Solid Edge part; units mm, degrees
sketch "Sketch1" plane through (0, 0, 0) normal (0, 0, 1) x (1, 0, 0)
  line L0 (-23, -6) -> (23, -6)
  arc A0 (23, 6) -> (23, -6) centre (23, 0) cw
  line L1 (23, 6) -> (-23, 6)
  arc A1 (-23, -6) -> (-23, 6) centre (-23, 0) cw
extrude "Protrusion1" add sketch "Sketch1" against normal blind 0.5
sketch "Sketch2" plane through (0, 0, 0) normal (0, 0, 1) x (1, 0, 0)
  circle A0 centre (26, 0) radius 1.5
extrude "ExtrudedProtrusion_2" add sketch "Sketch2" along normal blind 1
sketch "Sketch3" plane through (0, 0, 0) normal (0, 0, 1) x (1, 0, 0)
  line L0 (-12, -1.5) -> (20, -1.5)
  line L1 (20, -1.5) -> (20, 1.5)
  line L2 (20, 1.5) -> (-12, 1.5)
  line L3 (-12, -1.5) -> (-12, 1.5)
extrude "ExtrudedCutout_1" cut sketch "Sketch3" against normal blind 0.5
sketch "Sketch4" plane through (0, 0, 0) normal (0, 0, 1) x (1, 0, 0)
  circle A0 centre (-23, 3) radius 1
extrude "ExtrudedCutout_2" cut sketch "Sketch4" against normal blind 0.5
sketch "Sketch5" plane through (0, 0, 0) normal (0, 0, 1) x (1, 0, 0)
  circle A0 centre (-23, -3) radius 1
extrude "ExtrudedCutout_3" cut sketch "Sketch5" against normal blind 0.5
sketch "Sketch6" plane through (0, 0, 0) normal (0, 0, 1) x (1, 0, 0)
  circle A0 centre (23, 3) radius 1
extrude "ExtrudedCutout_4" cut sketch "Sketch6" against normal blind 0.5
sketch "Sketch7" plane through (0, 0, 0) normal (0, 0, 1) x (1, 0, 0)
  circle A0 centre (23, -3) radius 1
extrude "ExtrudedCutout_5" cut sketch "Sketch7" against normal blind 0.5
The listing builds one solid part. Answer for the finished solid, in the listing's coordinates (mm). Round coordinates to 2 decimals unless told otherwise and drop trailing zeros. Write each loop counter-clockwise with the first axis right and the second up, starting at its lowest first coordinate (ties: lowest second). Pieces come first, ordered by that corner, then holes. Notation, with made-up numbers: M 85.5,-33 L 97.5,-33 A9 cw 97.5,-29 Z; hole C 79.5,66 d5. An arc over 180 degrees is marked long. Write each question's results on one line, items separated by ' | '. Start each with the question number.
Item 1: Find section C-C on y = -0.5. Write down the section's boundary in (x, z), and give its area (3 significant figures).
Item 2: The mould has two halves that part along X. Classify faces 1 (the flat face through (0, 3, 0)), 2 (the cylindrical face through (-24, -3, -0.2)), 3 (the cylindrical face through (24.5, -0.07, 0.49)): +X half, -X half, draft (parallel to the pull), parting line (faces both ways), or undercut.
Item 3: Given pin 1 Ø6 at (x, y) = (19.5, 2.5) entering from +Z; pin 2 Ø1.8 at (x, y) = (23, 3) entering from -Z, each flat-ended and moving along its own axis, determine where each tip first touches the part or whether it passes through.
Item 4: Find section D-D on y = 3. Write down the section's boundary in (x, z).
Item 5: Find section A-A on x = 0. Write down the section's boundary in (y, z).
Item 6: Find section B-B on z = -0.25. Write down the section's boundary in (x, y), and give its area (3 significant figures).
Item 7: Straight lines are drawn through the part: probe 1 along Y at (x, z) = (-23, -0.1); probe 2 along Y at (x, z) = (3, -0.15); probe 3 along Z at (x, y) = (13, 3). For each, find the intervals that lie inside material, in ascending order.
Answer block:
1) outline: M -28.98,-0.5 L -12,-0.5 L -12,0 L -28.98,0 Z; M 20,-0.5 L 28.98,-0.5 L 28.98,0 L 27.41,0 L 27.41,1 L 24.59,1 L 24.59,0 L 20,0 Z | area: 15.8 mm²
2) face 1: draft | face 2: undercut | face 3: parting line
3) pin 1: stops at z = 0 | pin 2: passes through
4) outline: M -28.2,-0.5 L -24,-0.5 L -24,0 L -28.2,0 Z; M -22,-0.5 L 22,-0.5 L 22,0 L -22,0 Z; M 24,-0.5 L 28.2,-0.5 L 28.2,0 L 24,0 Z
5) outline: M -6,-0.5 L -1.5,-0.5 L -1.5,0 L -6,0 Z; M 1.5,-0.5 L 6,-0.5 L 6,0 L 1.5,0 Z
6) outline: M -23,-6 L 23,-6 A6 ccw 23,6 L -23,6 A6 ccw Z; hole C -23,-3 d2; hole C -23,3 d2; hole M -12,-1.5 L 20,-1.5 L 20,1.5 L -12,1.5 Z; hole C 23,-3 d2; hole C 23,3 d2 | area: 557 mm²
7) probe 1: y = -6 to -4, -2 to 2, 4 to 6 | probe 2: y = -6 to -1.5, 1.5 to 6 | probe 3: z = -0.5 to 0
